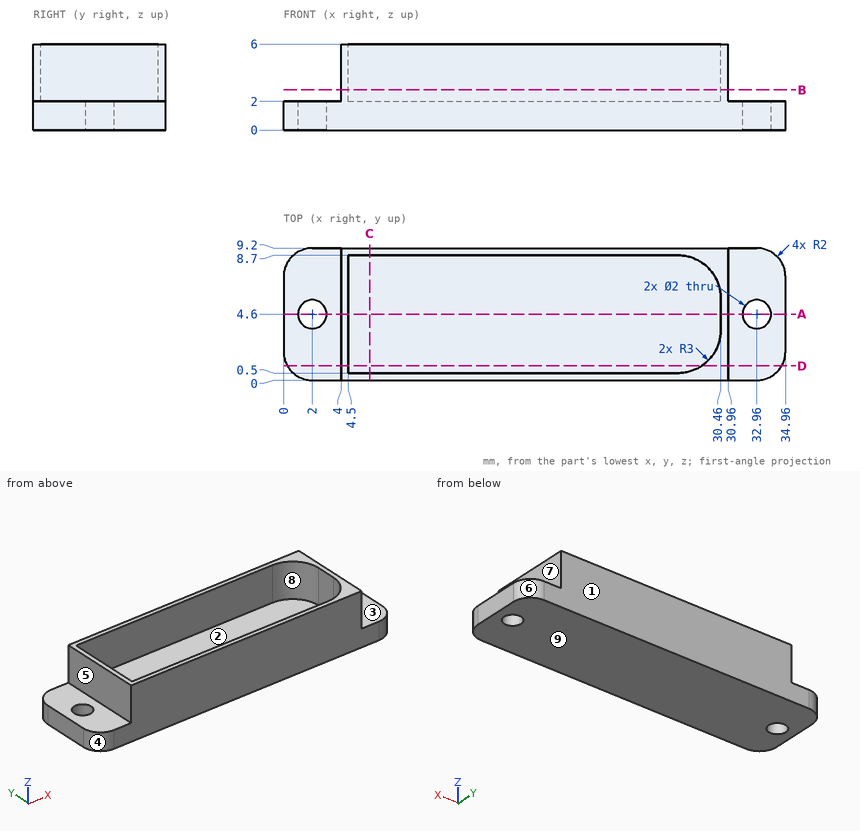
Part print with two shaded views. Sizes in mm from the minimum x, y, z corner. A direction names the side the tool comes from. Round coordinates to 2 decimals unless told otherwise and drop trailing zeros. Order: outer loops, then holes, each group sorted by start corner. A loop starts at its lowest first (then second) coordinate and runs counter-clockwise, first axis right, second up.
(1) 3-axis set-ups, long thin cutter, end or side, ignore diameter. For the marked faces 5, 6, 7, 8 and 9: which of +Z, -Z, +X, -X, +Y, -Y reach the whole face in a straight line?
(2) Pin check, flat tips, straight feed: pin 1 (1.2 mm diameter, centred on x = 33.5, y = 4, fed in from +Z); pin 2 (2 mm diameter, centred on y = 5, z = 3.5, fed in from -X); pin 3 (1.2 mm diameter, centred on y = 5, z = 4, fed in from +X). Stop position of each tip, or through.
(3) Band-saw the part on B-B (z = 2.8). List the corners of the cut face in (x, y), then the cut area to 3 significant figures.
(4) Band-saw the part on D-D (y = 1). List the corners of the cut face in (x, z).
(5) Drill centre lines: line 1 (Y direction, x = 32.96, z = 0.85); line 2 (Y direction, x = 22.5, z = 4.1); line 3 (X direction, y = 4.5, z = 1.65). Where is each one in solid material? Low to high.
(6) Band-saw the part on A-A (y = 4.6). List the corners of the cut face in (x, z).
(7) Band-saw the part on C-C (x = 6). List the corners of the cut face in (y, z), then the cut area to 3 significant figures.
(8) Pull direction Y, two halves, no side cores. Call the marked faces 1, 2, 3 and 4: released by +Y, released by -Y, zero draft, split by the parting line, or undercut.
Verdict:
1. face 5: +Z, -X, +Y, -Y
1. face 6: +Z, -Z, +X, +Y
1. face 7: +Z, +X, +Y, -Y
1. face 8: +Z
1. face 9: -Z, +X, -X, +Y, -Y
2. pin 1: stops at z = 2
2. pin 2: stops at x = 4
2. pin 3: stops at x = 30.96
3. outline: (4, 0) - (30.96, 0) - (30.96, 9.2) - (4, 9.2) - close; hole (4.5, 0.5) - (27.46, 0.5) arc R3 ccw to (30.46, 3.5) - (30.46, 5.7) arc R3 ccw to (27.46, 8.7) - (4.5, 8.7) - close
3. area: 39.0 mm2
4. outline: (0.27, 0) - (34.69, 0) - (34.69, 2) - (30.96, 2) - (30.96, 6) - (29.12, 6) - (29.12, 2) - (4.5, 2) - (4.5, 6) - (4, 6) - (4, 2) - (0.27, 2) - close
5. line 1: y = 0 to 3.6, 5.6 to 9.2
5. line 2: y = 0 to 0.5, 8.7 to 9.2
5. line 3: x = 0 to 1.01, 2.99 to 31.97, 33.95 to 34.96
6. outline: (0, 0) - (1, 0) - (1, 2) - (0, 2) - close; (3, 0) - (31.96, 0) - (31.96, 2) - (30.96, 2) - (30.96, 6) - (30.46, 6) - (30.46, 2) - (4.5, 2) - (4.5, 6) - (4, 6) - (4, 2) - (3, 2) - close; (33.96, 0) - (34.96, 0) - (34.96, 2) - (33.96, 2) - close
7. outline: (0, 0) - (9.2, 0) - (9.2, 6) - (8.7, 6) - (8.7, 2) - (0.5, 2) - (0.5, 6) - (0, 6) - close
7. area: 22.4 mm2
8. face 1: released by +Y
8. face 2: undercut
8. face 3: zero draft
8. face 4: released by -Y
